Job drawing, mm, ordinate dimensions from the low corner. One solid piece. A direction names the side the tool comes from. Give positions to 0.01 mm unless a question says otherwise; leave off trailing zeros. Write each loop counter-clockwise with the first axis right and the second up, starting at its lowest first coordinate (ties: lowest second). Pieces come first, ordered by that corner, then holes. Notation, with made-up numbers: (72, 10.25) - (93, 10.25) arc R30 cw to (93, 43.25) - close; hole circle Ø3 at (64.5, -12.75). An arc over 180 degrees is marked (long way). Answer as a JSON object with one key per item and string values.
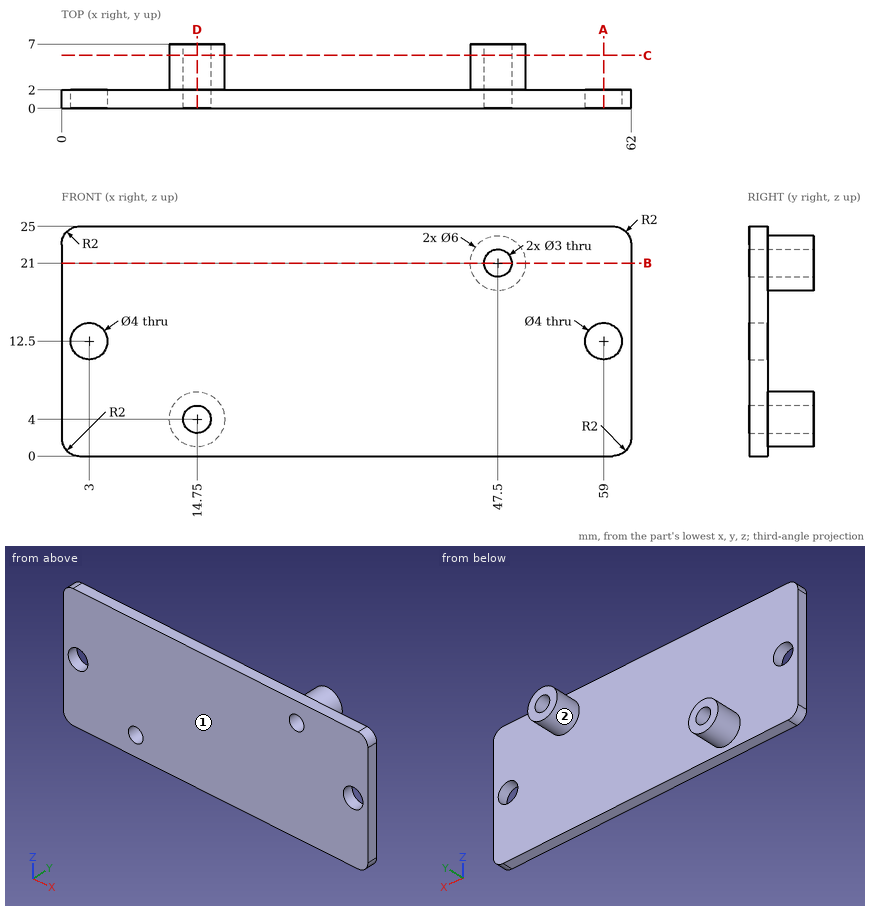
Item 1: Cut at A-A (x = 59). Give the cut face in (y, z).
Entries:
{"outline": "(0, 0) - (2, 0) - (2, 10.5) - (0, 10.5) - close; (0, 14.5) - (2, 14.5) - (2, 25) - (0, 25) - close"}
Item 2: Probe line 1 (X direction, y = 1.25, z = 12.5); line 2 (Z direction, x = 14.75, y = 2.25); line 3 (Z direction, x = 47.5, y = 3.25). List the from-to ranges inside material, lowest first. Write a range as from..to.
Entries:
{"line 1": "0..1, 5..57, 61..62", "line 2": "1..2.5, 5.5..7", "line 3": "18..19.5, 22.5..24"}
Item 3: Flat gauge pins, fed straight in: P1, Ø1.5, axis at y = 4, z = 3, coming from the +X side; P2, Ø5, axis at x = 3, z = 12.5, coming from the +Y side. Where does each tip first touch, or does it go through?
Entries:
{"P1": "x = 17.74", "P2": "y = 2"}
Item 4: Which spindle directions (+Z, -Z, +X, -X, +Y, -Y) get a long thin tool onto all of the face, cutting with end or side? Do the marked faces 1 and 2. Say none if no direction does.
Entries:
{"face 1": "+Z, -Z, +X, -X, -Y", "face 2": "+Y"}
Item 5: Cut at D-D (x = 14.75). Give the cut face in (y, z).
Entries:
{"outline": "(0, 0) - (2, 0) - (2, 1) - (7, 1) - (7, 2.5) - (0, 2.5) - close; (0, 5.5) - (7, 5.5) - (7, 7) - (2, 7) - (2, 25) - (0, 25) - close"}
Item 6: Cut at B-B (z = 21). Give the cut face in (x, y), and give its area (3 significant figures).
Entries:
{"outline": "(0, 0) - (46, 0) - (46, 7) - (44.5, 7) - (44.5, 2) - (0, 2) - close; (49, 0) - (62, 0) - (62, 2) - (50.5, 2) - (50.5, 7) - (49, 7) - close", "area": "133 mm2"}
Item 7: Cut at C-C (y = 5.75). Give the cut face in (x, z).
Entries:
{"outline": "circle Ø6 at (14.75, 4); circle Ø6 at (47.5, 21); hole circle Ø3 at (14.75, 4); hole circle Ø3 at (47.5, 21)"}
